```python
from build123d import *

# Parameters (mm, degrees)
BOX006_W               = 14
BOX006_H               = 8
BOX006_DEPTH           = 8.6
CYLINDER006_R          = 4.3
CYLINDER006_DEPTH      = 8
CYLINDER006_ROLL_ANGLE = 90
CYLINDER005_R          = 7.5
CYLINDER005_DEPTH      = 8
CYLINDER005_ROLL_ANGLE = 90
BOX005_W               = 14
BOX005_H               = 8
BOX005_DEPTH           = 8.6
BOX004_W               = 14
BOX004_H               = 8
BOX004_DEPTH           = 15.5
BOX_W                  = 48
BOX_H                  = 8
BOX_DEPTH              = 2


with BuildPart() as cubo006:
    # Box006 → Box006 (new body)
    with BuildSketch(Plane(origin=(-9, 0, 3.7), x_dir=(1, 0, 0), z_dir=(0, 0, 1))):
        with Locations((7, 4)):
            Rectangle(BOX006_W, BOX006_H)
    extrude(amount=BOX006_DEPTH)


with BuildPart() as cilindro006:
    # Cylinder006 → Cylinder006 (new body)
    with BuildSketch(Plane.XY):
        Circle(CYLINDER006_R)
    extrude(amount=CYLINDER006_DEPTH)


with BuildPart() as cilindro006_1:
    # Cylinder006 roll: moved
    add(cilindro006.part.rotate(Axis((0, 0, 0), (1, 0, 0)), CYLINDER006_ROLL_ANGLE))


with BuildPart() as cilindro006_2:
    # Cylinder006 placement: moved
    add(cilindro006_1.part.moved(Location((5, 8, 8))))


with BuildPart() as cut:
    # Cylinder005 → Cylinder005 (new body)
    with BuildSketch(Plane.XY):
        Circle(CYLINDER005_R)
    extrude(amount=CYLINDER005_DEPTH)


with BuildPart() as cut_1:
    # Cylinder005 roll: moved
    add(cut.part.rotate(Axis((0, 0, 0), (1, 0, 0)), CYLINDER005_ROLL_ANGLE))


with BuildPart() as cut_2:
    # Cylinder005 placement: moved
    add(cut_1.part.moved(Location((5, 8, 8))))

    # Cut004: cut Cilindro006
    add(cilindro006_2.part, mode=Mode.SUBTRACT)

    # Cut: cut Cubo006
    add(cubo006.part, mode=Mode.SUBTRACT)


with BuildPart() as cubo005:
    # Box005 → Box005 (new body)
    with BuildSketch(Plane(origin=(-9, 0, 3.7), x_dir=(1, 0, 0), z_dir=(0, 0, 1))):
        with Locations((7, 4)):
            Rectangle(BOX005_W, BOX005_H)
    extrude(amount=BOX005_DEPTH)


with BuildPart() as cut003:
    # Box004 → Box004 (new body)
    with BuildSketch(Plane(origin=(-9, 0, 0), x_dir=(1, 0, 0), z_dir=(0, 0, 1))):
        with Locations((7, 4)):
            Rectangle(BOX004_W, BOX004_H)
    extrude(amount=BOX004_DEPTH)

    # Cut003: cut Cubo005
    add(cubo005.part, mode=Mode.SUBTRACT)


with BuildPart() as fusion:
    # Box → Box (new body)
    with BuildSketch(Plane(origin=(-9, 0, 0), x_dir=(1, 0, 0), z_dir=(0, 0, 1))):
        with Locations((24, 4)):
            Rectangle(BOX_W, BOX_H)
    extrude(amount=BOX_DEPTH)

    # Fusion001003: union Cut003
    add(cut003.part)

    # Fusion: union Cut
    add(cut_2.part)


solid = fusion.part
```
The model under review builds one solid part; all positions refer to its coordinate system, in mm. A direction names the side the tool comes from. Round coordinates to 2 decimals unless told otherwise and drop trailing zeros. Loops run counter-clockwise (first coordinate to the right, second up) from the corner with the lowest first, then second, coordinate; pieces in that order, holes last. Notation, with made-up numbers: (82, 59) - (139, 59) arc R7 ccw to (139, 66) - close; hole circle Ø2 at (24.5, -37). An arc over 180 degrees is marked (long way). Use a Markdown table: item, result. Add a question column.
Q1. Add section A-A (x = -2). State the section outline as (y, z) points.
Q2. Add section C-C (x = 24.5). State the section outline as (y, z) points, plus the area to 3 significant figures.
Q3. Add section D-D (z = 8). State the section outline as (x, y) points, plus the area to 3 significant figures.
Q4. The part is to be moulded in two halves that separate along Z. For faces 3 (the face through (12.156, 4.056, 10.247)), 4 (the face through (9.3, 4.1, 7.9)), 5 (the face through (8, 8, 4)), 6 (the face through (15, 4, 0)), say which applies: pulls with the +Z half, pulls with the -Z half, needs draft (parallel to the pull), parting line crosses it, or undercut.
Q5. Add section B-B (y = 2). State the section outline as (x, z) points, plus the area to 3 significant figures.
Q6. For probe 1 along Z at (x, y) = (-2, 6.75); probe 2 along Z at (x, y) = (32, 3.75); probe 3 along Z at (x, y) = (6, 0.75), list the stretches that pass through material, from the lowest coordinate up.
Q7. Machinability: for faces 1 (the face through (-2, 4, 12.3)), 2 (the face through (-2, 4, 15.5)), which of the approach directions +Z, -Z, +X, -X, +Y, -Y give a long, thin tool a straight path to every point of the face, cutting with its end or side? Answer none if there is none.
Worked answers:
| question | item | result |
|---|---|---|
| 1 | outline | (0, 0) - (8, 0) - (8, 3.7) - (0, 3.7) - close; (0, 12.3) - (8, 12.3) - (8, 15.5) - (0, 15.5) - close |
| 2 | outline | (0, 0) - (8, 0) - (8, 2) - (0, 2) - close |
| 2 | area | 16.0 mm² |
| 3 | outline | (9.3, 0) - (12.5, 0) - (12.5, 8) - (9.3, 8) - close |
| 3 | area | 25.6 mm² |
| 4 | face 3 | undercut |
| 4 | face 4 | undercut |
| 4 | face 5 | needs draft |
| 4 | face 6 | pulls with the -Z half |
| 5 | outline | (-9, 0) - (39, 0) - (39, 2) - (9.5, 2) arc R7.5 ccw to (5, 15.5) - (-9, 15.5) - (-9, 12.3) - (5, 12.3) arc R4.3 cw to (5, 3.7) - (-9, 3.7) - close |
| 5 | area | 219 mm² |
| 6 | probe 1 | 0 to 3.7, 12.3 to 15.5 |
| 6 | probe 2 | 0 to 2 |
| 6 | probe 3 | 0 to 3.82, 12.18 to 15.43 |
| 7 | face 1 | -X, +Y, -Y |
| 7 | face 2 | +Z, +X, -X, +Y, -Y |
